```python
from build123d import *

# Parameters (mm, degrees)
BOSS_EXTRUDE1_DEPTH            = 38.1
FILLET1_R                      = 2.54
SKETCH3_R                      = 2.38125
GUESS_OF_WHERE_HOLES_ARE_DEPTH = 53.521397544
SKETCH4_R                      = 2.38125
CUT_EXTRUDE2_DEPTH             = 53.521397544


with BuildPart() as part:
    # Sketch2 → Boss-Extrude1 (new body)
    with BuildSketch(Plane(origin=(0, 0, 0), x_dir=(0, 0, -1), z_dir=(1, 0, 0))):
        Polygon((0, 0), (27.94, 0), (27.94, 5), (5, 5), (5, 27.94), (0, 27.94), align=None)
    extrude(amount=BOSS_EXTRUDE1_DEPTH)

    # Fillet1
    fillet1_edges = [part.edges().sort_by_distance(p)[0] for p in [
        (19.05, 5, -5),
        (19.05, 0, 0),
        (38.1, 2.5, -27.94),
        (0, 2.5, -27.94),
        (0, 27.94, -2.5),
        (38.1, 27.94, -2.5),
    ]]
    fillet(fillet1_edges, radius=FILLET1_R)

    # Sketch3 → guess_of_where_holes_are (cut, through all)
    with BuildSketch(Plane(origin=(0, 0, -5), x_dir=(-1, 0, 0), z_dir=(0, 0, -1))):
        with Locations((-31.75, 22.78)):
            Circle(SKETCH3_R)
        with Locations((-6.35, 22.78)):
            Circle(SKETCH3_R)
    extrude(amount=-GUESS_OF_WHERE_HOLES_ARE_DEPTH, mode=Mode.SUBTRACT)

    # Sketch4 → Cut-Extrude2 (cut, through all)
    with BuildSketch(Plane(origin=(0, 5, 0), x_dir=(1, 0, 0), z_dir=(0, 1, 0))):
        with Locations(Location((31.75, 22.78, 0), (0, 0, 270))):
            Circle(SKETCH4_R)
        with Locations(Location((6.35, 22.78, 0), (0, 0, 270))):
            Circle(SKETCH4_R)
    extrude(amount=-CUT_EXTRUDE2_DEPTH, mode=Mode.SUBTRACT)


solid = part.part
```
Geometry check sheet. Reference: the model listing, model coordinates, mm. A direction names the side the tool comes from. Give positions to 0.01 mm unless a question says otherwise; leave off trailing zeros. Order: outer loops, then holes, each group sorted by start corner. A loop starts at its lowest first (then second) coordinate and runs counter-clockwise, first axis right, second up.
1. Section check C-C, the plane x = 14.5. Enter the section's corners in (y, z), and give its area (3 significant figures).
2. Section check A-A, the plane x = 6.35. Enter the section's corners in (y, z), and give its area (3 significant figures).
3. Thickness scan on L1, parallel to Y at x = 31.75, z = -2.8; L2, parallel to X at y = 4, z = -22.25; L3, parallel to Z at x = 24.5, y = 9.25. Record the ranges inside material, lowest first.
4. Release check for a two-part mould opening along Z. For faces 1 (the face through (19.317, 0.724, -0.764)), 2 (the face through (0.764, 2.535, -27.216)), 3 (the face through (6.45, 2.54, -25.16)), 4 (the face through (34.11, 2.54, -23.09)) record: pulls with the +Z half, pulls with the -Z half, needs draft (parallel to the pull), parting line crosses it, or undercut.
5. Section check D-D, the plane z = -22.5. Enter the section's corners in (x, y).
6. Access from +Z, -Z, +X, -X, +Y, -Y to the whole of each face (thin tool, end or side, straight path). Record for faces 5 (the face through (5.25, 20.67, -2.54)), 6 (the face through (19, 5, -18)).
7. Section check B-B, the plane y = 22.78. Enter the section's corners in (x, z).
8. Gauge pin test, flat ends, axial feed: pin 1 Ø1.5 at (x, z) = (23, -10) entering from +Y; pin 2 Ø3 at (x, z) = (21.5, -8) entering from +Y. Record the tip position at first contact, or that the pin passes through.
Values follow:
1. outline: (0, -27.94) - (5, -27.94) - (5, -7.54) arc R2.54 cw to (7.54, -5) - (27.94, -5) - (27.94, 0) - (2.54, 0) arc R2.54 ccw to (0, -2.54) - close
1. area: 254 mm2
2. outline: (0, -27.94) - (5, -27.94) - (5, -25.16) - (0, -25.16) - close; (0, -20.4) - (5, -20.4) - (5, -7.54) arc R2.54 cw to (7.54, -5) - (20.4, -5) - (20.4, 0) - (2.54, 0) arc R2.54 ccw to (0, -2.54) - close; (25.16, -5) - (27.94, -5) - (27.94, 0) - (25.16, 0) - close
2. area: 207 mm2
3. L1: y = 0 to 20.4, 25.16 to 27.94
3. L2: x = 0 to 4.03, 8.67 to 29.43, 34.07 to 38.1
3. L3: z = -5 to 0
4. face 1: pulls with the +Z half
4. face 2: pulls with the -Z half
4. face 3: undercut
4. face 4: undercut
5. outline: (0, 0) - (3.99, 0) - (3.99, 5) - (0, 5) - close; (8.71, 0) - (29.39, 0) - (29.39, 5) - (8.71, 5) - close; (34.11, 0) - (38.1, 0) - (38.1, 5) - (34.11, 5) - close
6. face 5: +Z, -Z
6. face 6: -Z, +X, -X, +Y
7. outline: (0, -5) - (3.97, -5) - (3.97, 0) - (0, 0) - close; (8.73, -5) - (29.37, -5) - (29.37, 0) - (8.73, 0) - close; (34.13, -5) - (38.1, -5) - (38.1, 0) - (34.13, 0) - close
8. pin 1: stops at y = 5
8. pin 2: stops at y = 5.22
